```python
from build123d import *

# Parameters (mm, degrees)
F1_R     = 2.75
F1_R_2   = 2
F2_DEPTH = 4.2
F4_DEPTH = 1.6


with BuildPart() as f2:
    # F1 (on Front) → F2 (new body)
    with BuildSketch(Plane.XZ):
        with BuildLine():
            Line((-6.3493797847, -4), (-6.3493798562, 27.98366989))
            ThreePointArc((-6.3493798562, 27.98366989), (-11.3493798562, 32.9836699012), (-16.3493798562, 27.98366989))
            Line((-16.3493798562, 27.98366989), (-16.3493798515, 25.8790112235))
            Line((-16.3493798515, 25.8790112235), (-22.9881312178, 23.98366989))
            Line((-22.9881312178, 23.98366989), (-16.3493798405, 20.9362090031))
            Line((-16.3493798405, 20.9362090031), (-16.3493797847, -4))
            ThreePointArc((-16.3493797847, -4), (0, -20.349379785), (16.3493797847, -4))
            Line((16.3493797847, -4), (16.3493797847, 0))
            ThreePointArc((16.3493797847, 0), (11.3493797847, 5), (6.3493797847, 0))
            Line((6.3493797847, 0), (6.3493797847, -4))
            ThreePointArc((6.3493797847, -4), (0, -10.3493797847), (-6.3493797847, -4))
        make_face()
        with Locations((11.3493797847, 0)):
            Circle(F1_R, mode=Mode.SUBTRACT)
        with Locations((-11.3493798562, 27.9836699012)):
            Circle(F1_R_2, mode=Mode.SUBTRACT)
    extrude(amount=F2_DEPTH)

    # F3 (on face) → F4 (cut)
    with BuildSketch(Plane.XZ.offset(4.2)):
        with BuildLine():
            ThreePointArc((9.8993797847, -2.3366642891), (11.3493797847, -2.75), (12.7993797847, -2.3366642891))
            ThreePointArc((12.7993797847, -2.3366642891), (13.7525027528, -1.3369741957), (14.0993797847, 0))
            ThreePointArc((14.0993797847, 0), (10.012405589, 2.4031229681), (9.8993797847, -2.3366642891))
        make_face()
        with BuildLine():
            Line((12.7993797847, -5.05), (12.7993797847, -2.3366642891))
            ThreePointArc((12.7993797847, -2.3366642891), (11.3493797847, -2.75), (9.8993797847, -2.3366642891))
            Line((9.8993797847, -2.3366642891), (9.8993797847, -5.05))
            ThreePointArc((9.8993797847, -5.05), (11.3493797847, -6.5), (12.7993797847, -5.05))
        make_face()
    extrude(amount=-F4_DEPTH, mode=Mode.SUBTRACT)


solid = f2.part
```
Can you work these out from the model? Positions are in its coordinate system, mm. A direction names the side the tool comes from. Give positions to 0.01 mm unless a question says otherwise; leave off trailing zeros. Loops run counter-clockwise (first coordinate to the right, second up) from the corner with the lowest first, then second, coordinate; pieces in that order, holes last. Notation, with made-up numbers: M 5.5,-13.75 L 19.5,-13.75 A26 cw 19.5,20.25 Z; hole C 3.5,54 d7. An arc over 180 degrees is marked long. One line per item, written item: value.
(1) Suppose I cut it at C-C on x = 0. List the corners of the cut face in (y, z) for me, plus the area to 3 significant figures.
Returned:
outline: M -4.2,-20.35 L 0,-20.35 L 0,-10.35 L -4.2,-10.35 Z
area: 42.0 mm^2
(2) I need wall thicknesses on line 1 (Z direction, x = 0, y = -2.75); line 2 (X direction, y = -2.45, z = -0.5); line 3 (X direction, y = -0.45, z = -2). Which ranges of each line are inside material? Lowest first, please.
Returned:
line 1: -20.35 to -10.35
line 2: -16.35 to -6.35, 6.35 to 8.65, 14.05 to 16.35
line 3: -16.35 to -6.35, 6.35 to 9.46, 13.24 to 16.35
(3) Suppose I cut it at B-B on x = 11. List the corners of the cut face in (y, z) for me.
Returned:
outline: M -4.2,-16.1 L 0,-16.1 L 0,-2.73 L -2.6,-2.73 L -2.6,-6.46 L -4.2,-6.46 Z; M -4.2,2.73 L 0,2.73 L 0,4.99 L -4.2,4.99 Z
(4) Suppose I cut it at A-A on y = -3.25. List the corners of the cut face in (x, z) for me, plus the area to 3 significant figures.
Returned:
outline: M -22.99,23.98 L -16.35,20.94 L -16.35,-4 A16.35 ccw 16.35,-4 L 16.35,0 A5 ccw 6.35,0 L 6.35,-4 A6.35 cw -6.35,-4 L -6.35,27.98 A5 ccw -16.35,27.98 L -16.35,25.88 Z; hole C -11.35,27.98 d4; hole M 9.9,-5.05 A1.45 ccw 12.8,-5.05 L 12.8,-2.34 A2.75 ccw long 9.9,-2.34 Z
area: 765 mm^2
(5) Which directions (+Z, -Z, +X, -X, +Y, -Y) give clear straight access to the entire face, cutting with the end or side of a thin tool? Please do faces 5 (the face through (-16.349, -2, 9)), 6 (the face through (-16.349, -2, 27)), 7 (the face through (12.799, -3, -4)), 8 (the face through (6.349, -2, -2)).
Returned:
face 5: -Z, -X, +Y, -Y
face 6: +Z, -X, +Y, -Y
face 7: -Y
face 8: +Z, +Y, -Y
(6) Suppose I cut it at D-D on z = 15. List the corners of the cut face in (x, y) for me.
Returned:
outline: M -16.35,-4.2 L -6.35,-4.2 L -6.35,0 L -16.35,0 Z
(7) We'd pull the mould along X, two halves only. Please class faces 1 (the face through (16.349, -2, -2)), 2 (the face through (10.991, -2.071, 2.727)), 3 (the face through (-11.239, -2.071, 32.982)), 4 (the face through (9.899, -3, -4)): released by +X, released by -X, zero draft, split by the parting line, or undercut.
Returned:
face 1: released by +X
face 2: undercut
face 3: split by the parting line
face 4: undercut
(8) Will these pins go through, and if not, where does the flat tip stop? pin 1 (1.5 mm diameter, centred on y = -2, z = 10, fed in from -X); pin 2 (0.9 mm diameter, centred on x = 12, z = -4, fed in from -Y); pin 3 (2 mm diameter, centred on x = 9.5, y = -3.5, fed in from +Z).
Returned:
pin 1: x = -16.35
pin 2: y = -2.6
pin 3: z = 4.93
